Job drawing, mm, ordinate dimensions from the low corner. One solid piece. A direction names the side the tool comes from. Give positions to 0.01 mm unless a question says otherwise; leave off trailing zeros. Loops run counter-clockwise (first coordinate to the right, second up) from the corner with the lowest first, then second, coordinate; pieces in that order, holes last. Notation, with made-up numbers: M -27,-11.75 L 31,-11.75 A27 ccw 31,27.25 Z; hole C -10.75,-34.75 d9. An arc over 180 degrees is marked long. Put each result on its own line as item: value.
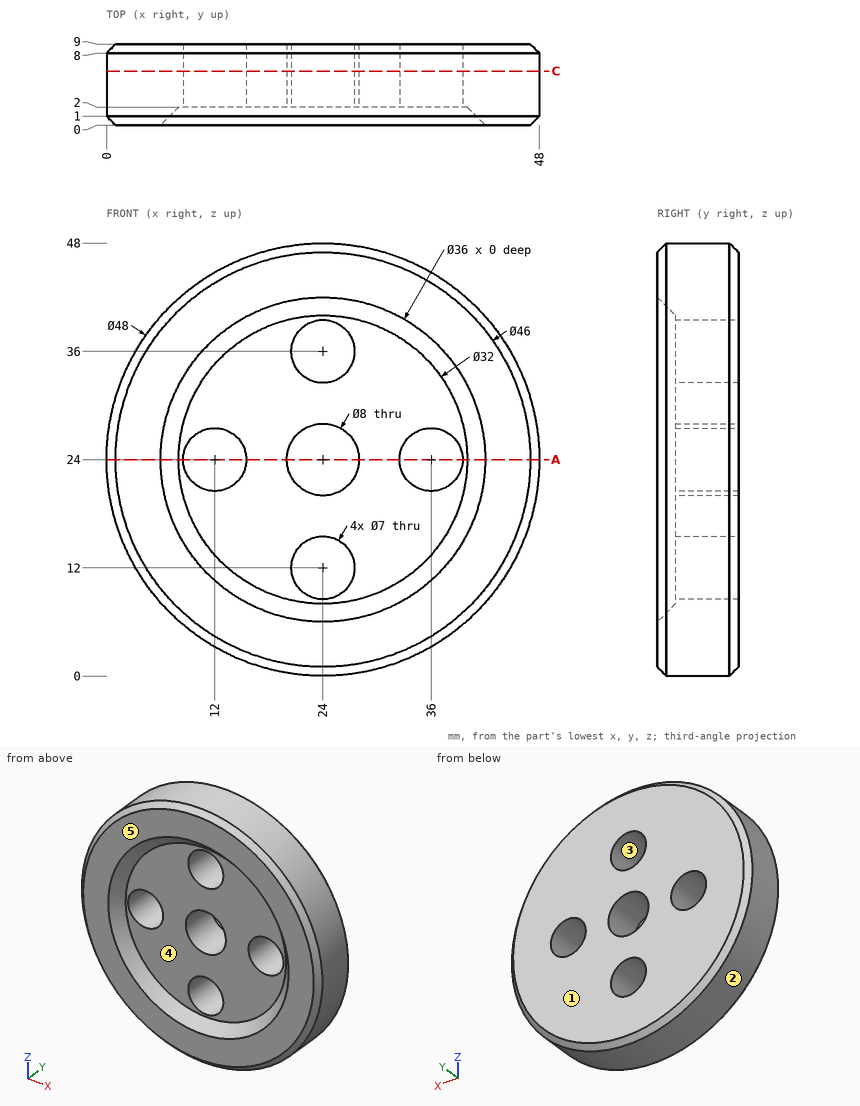
Q1. Slice it at A-A (z = 24). State how many separate pieces and enclosed holes the cut face has, and give its area (3 significant figures).
Here are the results:
separate pieces: 4
enclosed holes: 0
area: 208 mm²
Q2. Drop flat-ended pins along their axis: pin 1 Ø3 at (y, z) = (5, 26) entering from +X (3 decimals); pin 2 Ø4 at (x, y) = (43, 5.5) entering from +Z; pin 3 Ø9 at (x, z) = (24, 12) entering from -Y. Give the stop position or say it passes through.
Here are the results:
pin 1: x = 47.995
pin 2: z = 40.94
pin 3: y = 1.5
Q3. Mould opens along Z. For the marked faces 1, 2 and 3 say: pulls with the +Z half, pulls with the -Z half, needs draft (parallel to the pull), parting line crosses it, or undercut.
Here are the results:
face 1: needs draft
face 2: parting line crosses it
face 3: undercut
Q4. Probe line 1 (X direction, y = 5.25, z = 24); line 2 (Z direction, x = 21, y = 4) (1 decimal); line 3 (X direction, y = 5, z = 12) (1 decimal). List the from-to ranges inside material, lowest first. Write a range as from..to.
Here are the results:
line 1: 0..8.5, 15.5..20, 28..32.5, 39.5..48
line 2: 0.2..10.2, 13.8..21.4, 26.6..34.2, 37.8..47.8
line 3: 3.2..20.5, 27.5..44.8
Q5. Slice it at C-C (y = 6). List the corners of the cut face in (x, z), and give its area (3 significant figures).
Here are the results:
outline: C 24,24 d48; hole C 12,24 d7; hole C 24,24 d8; hole C 24,12 d7; hole C 24,36 d7; hole C 36,24 d7
area: 1,610 mm²
Q6. Tool access for the marked faces 4 and 5: list every direction of +Z, -Z, +X, -X, +Y, -Y with a clear straight run to the whole face (end or side of a thin tool).
Here are the results:
face 4: -Y
face 5: +Z, -Z, +X, -X, -Y
